```python
from build123d import *

# Parameters (mm, degrees)
ESQUISSE1_W                                        = 40
ESQUISSE1_H                                        = 80
BOSS_EXTRU_1_DEPTH                                 = 10
CHANFREIN1_SIZE                                    = 2
TROU_TARAUD_M61_D                                  = 5
CHAMBRAGE_POUR_VIS_T_TE_HEXAGONALE_M51_D           = 5.5
CHAMBRAGE_POUR_VIS_T_TE_HEXAGONALE_M51_CBORE_D     = 10
CHAMBRAGE_POUR_VIS_T_TE_HEXAGONALE_M51_CBORE_DEPTH = 7


with BuildPart() as part:
    # Esquisse1 → Boss.-Extru.1 (new body)
    with BuildSketch(Plane.XY):
        Rectangle(ESQUISSE1_W, ESQUISSE1_H)
    extrude(amount=BOSS_EXTRU_1_DEPTH)

    # Chanfrein1
    chanfrein1_edges = [part.edges().sort_by_distance(p)[0] for p in [
        (-20, 40, 5),
        (20, 40, 5),
        (20, -40, 5),
        (-20, -40, 5),
    ]]
    chamfer(chanfrein1_edges, length=CHANFREIN1_SIZE)

    # Trou taraudé M61 (through all)
    with Locations(Plane.XY.offset(10)):
        with Locations((8, 31.5), (8, -31.5)):
            Hole(TROU_TARAUD_M61_D / 2)

    # Chambrage pour vis à tête hexagonale M51 (through all)
    with Locations(Plane.XY.offset(10)):
        with Locations((10, 10), (-10, -10)):
            CounterBoreHole(CHAMBRAGE_POUR_VIS_T_TE_HEXAGONALE_M51_D / 2, CHAMBRAGE_POUR_VIS_T_TE_HEXAGONALE_M51_CBORE_D / 2, CHAMBRAGE_POUR_VIS_T_TE_HEXAGONALE_M51_CBORE_DEPTH)


solid = part.part
```
Work out the finished part from the listing and answer in its coordinate system (mm). A direction names the side the tool comes from. Coordinates: 2 decimals unless noted, no trailing zeros. Loops run counter-clockwise (first coordinate to the right, second up) from the corner with the lowest first, then second, coordinate; pieces in that order, holes last. Notation, with made-up numbers: (60, 55) - (72, 55) arc R19 ccw to (72, 75) - close; hole circle Ø3 at (42, -32.5). An arc over 180 degrees is marked (long way). Use a Markdown table: item, result.
Item 1: The mould has two halves that part along Y. Classify faces 1 (the flat face through (-19, 39, 5)), 2 (the cylindrical face through (-12.62, -9.17, 1.48)), 3 (the flat face through (19, -39, 5)): +Y half, -Y half, draft (parallel to the pull), parting line (faces both ways), or undercut.
Evaluation:
| item | result |
|---|---|
| face 1 | +Y half |
| face 2 | undercut |
| face 3 | -Y half |
Item 2: Given pin 1 Ø4.5 at (x, y) = (8, 31.5) entering from -Z; pin 2 Ø7 at (x, y) = (-10, -10) entering from +Z, each flat-ended and moving along its own axis, determine where each tip first touches the part or whether it passes through.
Evaluation:
| item | result |
|---|---|
| pin 1 | passes through |
| pin 2 | stops at z = 3 |
Item 3: Find section A-A, the plane y = 31.5. Determine the outline of the cut face in (x, z).
Evaluation:
| item | result |
|---|---|
| outline | (-20, 0) - (5.5, 0) - (5.5, 10) - (-20, 10) - close; (10.5, 0) - (20, 0) - (20, 10) - (10.5, 10) - close |
Item 4: Consider probe 1 along Y at (x, z) = (10, 0.7); probe 2 along Y at (x, z) = (10, 6); probe 3 along Y at (x, z) = (-10, 1.6). Determine where each line is inside the solid, lowest interval first. Write a range as from..to.
Evaluation:
| item | result |
|---|---|
| probe 1 | y = -40..-33, -30..7.25, 12.75..30, 33..40 |
| probe 2 | y = -40..-33, -30..5, 15..30, 33..40 |
| probe 3 | y = -40..-12.75, -7.25..40 |
Item 5: Find section D-D, the plane x = 9. Determine the outline of the cut face in (y, z).
Evaluation:
| item | result |
|---|---|
| outline | (-40, 0) - (-33.79, 0) - (-33.79, 10) - (-40, 10) - close; (-29.21, 0) - (7.44, 0) - (7.44, 3) - (5.1, 3) - (5.1, 10) - (-29.21, 10) - close; (12.56, 0) - (29.21, 0) - (29.21, 10) - (14.9, 10) - (14.9, 3) - (12.56, 3) - close; (33.79, 0) - (40, 0) - (40, 10) - (33.79, 10) - close |
Item 6: For faces 4 (the flat face through (0, 40, 5)), 5 (the cylindrical face through (-5.23, -8.5, 6.55)), determine the directions among +Z, -Z, +X, -X, +Y, -Y from which every point of the face is accessible in a straight line to the end or side of a thin tool.
Evaluation:
| item | result |
|---|---|
| face 4 | +Z, -Z, +X, -X, +Y |
| face 5 | +Z |
Item 7: Find section B-B, the plane x = -10. Determine the outline of the cut face in (y, z), and give its area (4 significant figures).
Evaluation:
| item | result |
|---|---|
| outline | (-40, 0) - (-12.75, 0) - (-12.75, 3) - (-15, 3) - (-15, 10) - (-40, 10) - close; (-7.25, 0) - (40, 0) - (40, 10) - (-5, 10) - (-5, 3) - (-7.25, 3) - close |
| area | 713.5 mm2 |
Item 8: Find section C-C, the plane z = 4.25. Determine the outline of the cut face in (x, y).
Evaluation:
| item | result |
|---|---|
| outline | (-20, -38) - (-18, -40) - (18, -40) - (20, -38) - (20, 38) - (18, 40) - (-18, 40) - (-20, 38) - close; hole circle Ø10 at (-10, -10); hole circle Ø10 at (10, 10); hole circle Ø5 at (8, -31.5); hole circle Ø5 at (8, 31.5) |
